Work out the finished part from the listing and answer in its coordinate system (mm). Face numbers are marked on the shaded views. Coordinates: 2 decimals unless noted, no trailing zeros. Loops run counter-clockwise (first coordinate to the right, second up) from the corner with the lowest first, then second, coordinate; pieces in that order, holes last. Notation, with made-up numbers: (-18, 0.5) - (-10, 0.5) arc R22 cw to (-10, 36.5) - close; hole circle Ø7 at (78.25, 28). An arc over 180 degrees is marked (long way). Write each question's results on one line, items separated by ' | '. Start each with the question number.
Item 1: Consider probe 1 along Y at (x, z) = (2.5, 4.25); probe 2 along X at (y, z) = (-4, 13.5); probe 3 along Y at (x, z) = (5.75, 3). Determine where each line is inside the solid, lowest interval first. Write a range as [from, to].
Item 2: Section A-A, the plane y = 6.75 is taken. Write down the section's boundary in (x, z), plus the area to 3 significant figures.
Item 3: For a pull along X with two mould halves and no side action, classify the marked faces 1, 2, 3 and 4 as +X half, -X half, draft (parallel to the pull), parting line (faces both ways), or undercut.
Item 4: Each of these flat-tipped pins is pushed along its axis until it touches: pin 1 Ø0.8 at (x, y) = (-3, 0.5) entering from -Z; pin 2 Ø7.5 at (y, z) = (-4.5, 5) entering from +X; pin 3 Ø4 at (x, y) = (8.5, -3) entering from -Z; pin 4 Ø3 at (y, z) = (0.5, 6) entering from +X. Where does it stop, or does it pass through?
from build123d import *

# Parameters (mm, degrees)
AUFSATZ_LINEAR_AUSTRAGEN1_DEPTH = 15
SKIZZE2_W                       = 15
SKIZZE2_H                       = 19
AUFSATZ_LINEAR_AUSTRAGEN2_DEPTH = 3
SCHNITT_LINEAR_AUSTRAGEN1_DEPTH = 2
SKIZZE5_W                       = 15
SKIZZE5_H                       = 19
AUFSATZ_LINEAR_AUSTRAGEN4_DEPTH = 0.5


# Read off the part's stored shape, not the designer's step: Aufsatz-Linear austragen1
with BuildPart() as part:
    # Aufsatz-Linear austragen1 outline → Aufsatz-Linear austragen1 (new body)
    with BuildSketch(Plane.XY):
        with BuildLine():
            Line((9, 7.5), (9, 5.971762746))
            add(Edge.make_bspline(
                [(9, 5.971762746), (0.820844208, -0.941876975), (6, -9.5)],
                knots=[0.100732064, 0.100732064, 0.100732064, 1, 1, 1], degree=2))
            Line((6, -9.5), (6.855533767, -8.982252983))
            add(Edge.make_bspline(
                [(11, 6.271626074), (10.77340825, 6.105599677), (10.141366733, 5.627846644), (8.84701886, 4.547968637), (7.334591853, 2.994846091), (6.045831159, 1.119520738), (5.251441489, -0.76880078), (4.926102544, -2.686703365), (5.056978024, -4.672427827), (5.564804841, -6.418461308), (6.213216116, -7.858576344), (6.635759495, -8.619102834), (6.855533767, -8.982252983)],
                knots=[0.028407204, 0.028407204, 0.028407204, 0.028407204, 0.0625, 0.125, 0.25, 0.375, 0.5, 0.625, 0.75, 0.875, 0.9375, 1, 1, 1, 1], degree=3))
            Line((11, 6.271626074), (11, 9.5))
            Line((11, 9.5), (-1, 9.5))
            Line((-1, 9.5), (-1, -9.5))
            Line((-1, -9.5), (1, -9.5))
            Line((1, -9.5), (1, 7.5))
            Line((1, 7.5), (9, 7.5))
        make_face()
    extrude(amount=AUFSATZ_LINEAR_AUSTRAGEN1_DEPTH)

    # Skizze2 → Aufsatz-Linear austragen2 (add)
    with BuildSketch(Plane.ZY.offset(1)):
        with Locations((7.5, 0)):
            Rectangle(SKIZZE2_W, SKIZZE2_H)
    extrude(amount=AUFSATZ_LINEAR_AUSTRAGEN2_DEPTH)

    # Skizze3 → Schnitt-Linear austragen1 (cut)
    with BuildSketch(Plane.ZY.offset(4)):
        with BuildLine():
            Line((4.25, -0.5), (4.25, 1))
            ThreePointArc((4.25, 1), (7.5, 4.25), (10.75, 1))
            Line((10.75, 1), (10.75, -0.5))
            ThreePointArc((10.75, -0.5), (7.5, -3.75), (4.25, -0.5))
        make_face()
    extrude(amount=-SCHNITT_LINEAR_AUSTRAGEN1_DEPTH, mode=Mode.SUBTRACT)

    # Skizze5 → Aufsatz-Linear austragen4 (add)
    with BuildSketch(Plane.ZY.offset(4)):
        with Locations((7.5, 0)):
            Rectangle(SKIZZE5_W, SKIZZE5_H)
    extrude(amount=-AUFSATZ_LINEAR_AUSTRAGEN4_DEPTH)


solid = part.part
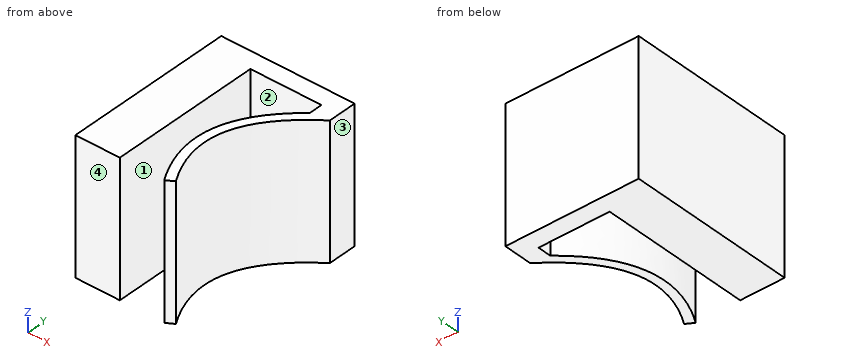
Answer key:
1) probe 1: y = [7.5, 9.5] | probe 2: x = [-4, 1], [4.03, 5.04] | probe 3: y = [-9.07, -6.79], [0.36, 2.42], [7.5, 9.5]
2) outline: (-4, 0) - (1, 0) - (1, 15) - (-4, 15) - close; (9, 0) - (11, 0) - (11, 15) - (9, 15) - close | area: 105 mm^2
3) face 1: undercut | face 2: undercut | face 3: +X half | face 4: draft
4) pin 1: stops at z = 0 | pin 2: stops at x = 6.44 | pin 3: passes through | pin 4: stops at x = 6.67
